Check sheet for the modelled part. Datum: model origin and axes. Units: mm. Give positions to 0.01 mm unless a question says otherwise; leave off trailing zeros. Loops run counter-clockwise (first coordinate to the right, second up) from the corner with the lowest first, then second, coordinate; pieces in that order, holes last. Notation, with made-up numbers: (37.25, 53.25) - (87.25, 53.25) arc R32 ccw to (87.25, 81.25) - close; hole circle Ø4 at (31.5, 81). An arc over 180 degrees is marked (long way). Answer in a Markdown table with one row per item. Add a question column.
(1) Sectioned sample at C-C on x = -3. Enter the section's corners in (y, z), then the cut area to 3 significant figures.
(2) Thickness scan on L1, parallel to Z at x = 1, y = -0.3; L2, parallel to Z at x = 3, y = -0.6; L3, parallel to X at y = -0.25, z = -1.75. Record the ranges inside material, lowest first.
(3) Sectioned sample at D-D on z = -6. Enter the section's corners in (x, y).
(4) Draft check along Z on faces 1 (the face through (7.4, -0.33, 7.33)), 2 (the face through (2, 0, 2)), 3 (the face through (1.6, -0.33, 1.66)). Enter one of: released by +Z, released by -Z, zero draft, split by the parting line, or undercut.
(5) Sectioned sample at B-B on y = -0.2. Enter the section's corners in (x, z), then the cut area to 3 significant figures.
(6) Sectioned sample at A-A on z = 3. Enter the section's corners in (x, y), then the cut area to 3 significant figures.
from build123d import *

# Parameters (mm, degrees)
F1_DEPTH = 0.67


with BuildPart() as f1:
    # F0 (on Front) → F1 (new body)
    with BuildSketch(Plane.XZ):
        with BuildLine():
            Line((3.83, 8.83), (-3.83, 8.83))
            ThreePointArc((-3.83, 8.83), (-7.365534, 7.365534), (-8.83, 3.83))
            Line((-8.83, 3.83), (-8.83, -3.83))
            ThreePointArc((-8.83, -3.83), (-7.365534, -7.365534), (-3.83, -8.83))
            Line((-3.83, -8.83), (3.83, -8.83))
            ThreePointArc((3.83, -8.83), (7.365534, -7.365534), (8.83, -3.83))
            Line((8.83, -3.83), (8.83, 3.83))
            ThreePointArc((8.83, 3.83), (7.365534, 7.365534), (3.83, 8.83))
        make_face()
        with BuildLine():
            ThreePointArc((4.643209, 0), (1.630041, -1.630041), (0, -4.643209))
            ThreePointArc((0, -4.643209), (-1.630041, -1.630041), (-4.643209, 0))
            ThreePointArc((-4.643209, 0), (-1.630041, 1.630041), (0, 4.643209))
            ThreePointArc((0, 4.643209), (1.630041, 1.630041), (4.643209, 0))
        make_face(mode=Mode.SUBTRACT)
    extrude(amount=F1_DEPTH)


solid = f1.part
Reply:
| question | item | result |
|---|---|---|
| 1 | outline | (-0.67, -8.83) - (0, -8.83) - (0, -0.61) - (-0.67, -0.61) - close; (-0.67, 0.61) - (0, 0.61) - (0, 8.83) - (-0.67, 8.83) - close |
| 1 | area | 11.0 mm^2 |
| 2 | L1 | -8.83 to -2.37, 2.37 to 8.83 |
| 2 | L2 | -8.83 to -0.61, 0.61 to 8.83 |
| 2 | L3 | -8.83 to -1.51, 1.51 to 8.83 |
| 3 | outline | (-8.33, -0.67) - (8.33, -0.67) - (8.33, 0) - (-8.33, 0) - close |
| 4 | face 1 | released by +Z |
| 4 | face 2 | zero draft |
| 4 | face 3 | undercut |
| 5 | outline | (-8.83, -3.83) arc R5 ccw to (-3.83, -8.83) - (3.83, -8.83) arc R5 ccw to (8.83, -3.83) - (8.83, 3.83) arc R5 ccw to (3.83, 8.83) - (-3.83, 8.83) arc R5 ccw to (-8.83, 3.83) - close; hole (-4.64, 0) arc R6 cw to (0, -4.64) arc R6 cw to (4.64, 0) arc R6 cw to (0, 4.64) arc R6 cw to start |
| 5 | area | 265 mm^2 |
| 6 | outline | (-8.83, -0.67) - (-0.61, -0.67) - (-0.61, 0) - (-8.83, 0) - close; (0.61, -0.67) - (8.83, -0.67) - (8.83, 0) - (0.61, 0) - close |
| 6 | area | 11.0 mm^2 |
